from build123d import *

# Parameters (mm, degrees)
F0_W     = 15
F0_H     = 26.12
F0_W_2   = 112.35
F0_H_2   = 29.4448914682
F0_W_3   = 37.3
F1_DEPTH = 100
F2_R     = 5
F3_R     = 1
F4_R     = 0.49999
F5_R     = 3


# Not quite as in the source:
# - two fillets or chamfers of one size are made in one step
# - a fillet or chamfer is up to 0.001 mm smaller than in the source, because OpenCascade refuses the exact size
# - a feature names something its author has since deleted; it is built from what else it names


with BuildPart() as f1:
    # F0 (on Front) → F1 (new body)
    with BuildSketch(Plane.XZ):
        Polygon((0, 141.95), (0, 0), (23, 0), (23, -2), (25, -2), (25, 0), (48.9, 0), (48.9, 13.7202170637), (99.9, 13.7202170637), (99.9, 30.4702170637), (178.65, 30.4702170637), (178.65, 95.36), (28, 95.36), (28, 141.95), align=None)
        with Locations((12.5, 15.06)):
            Rectangle(F0_W, F0_H, mode=Mode.SUBTRACT)
        Polygon((25, 2), (25, 28.12), (46.9, 14.6043096234), (46.9, 2), align=None, mode=Mode.SUBTRACT)
        Polygon((97.9, 15.7202170637), (48.9, 15.7202170637), (25, 30.4702170637), (97.9, 30.4702170637), align=None, mode=Mode.SUBTRACT)
        with Locations((12.5, 46.18)):
            Rectangle(F0_W, F0_H, mode=Mode.SUBTRACT)
        with Locations((81.175, 47.1926627978)):
            Rectangle(F0_W_2, F0_H_2, mode=Mode.SUBTRACT)
        with Locations((158, 47.1926627978)):
            Rectangle(F0_W_3, F0_H_2, mode=Mode.SUBTRACT)
        with Locations((12.5, 77.3)):
            Rectangle(F0_W, F0_H, mode=Mode.SUBTRACT)
        with Locations((81.175, 78.6375542659)):
            Rectangle(F0_W_2, F0_H_2, mode=Mode.SUBTRACT)
        Polygon((25, 95.36), (5, 95.36), (5, 138.95), (17, 138.95), (17, 139.95), (25, 139.95), align=None, mode=Mode.SUBTRACT)
        with Locations((158, 78.6375542659)):
            Rectangle(F0_W_3, F0_H_2, mode=Mode.SUBTRACT)
    extrude(amount=F1_DEPTH)

    # F2
    f2_edges = [f1.edges().sort_by_distance(p)[0] for p in [
        (28, -50, 95.36),
        (25, -50, 28.12),
        (25, -50, 32.470217),
        (25, -50, 61.915109),
        (25, -50, 93.36),
        (25, -50, 63.915109),
    ]]
    fillet(f2_edges, radius=F2_R)

    # F3
    f3_edges = [f1.edges().sort_by_distance(p)[0] for p in [
        (5, -50, 64.24),
        (5, -50, 33.12),
        (5, -50, 2),
        (5, -50, 90.36),
        (5, -50, 59.24),
        (5, -50, 28.12),
        (20, -50, 28.12),
        (20, -50, 59.24),
        (20, -50, 90.36),
        (20, -50, 64.24),
        (20, -50, 33.12),
        (20, -50, 2),
        (46.9, -50, 2),
        (46.9, -50, 14.60431),
        (25, -50, 30.470217),
        (97.9, -50, 15.720217),
        (97.9, -50, 30.470217),
        (137.35, -50, 61.915109),
        (137.35, -50, 93.36),
        (137.35, -50, 63.915109),
        (137.35, -50, 32.470217),
        (176.65, -50, 32.470217),
        (176.65, -50, 63.915109),
        (139.35, -50, 63.915109),
        (139.35, -50, 61.915109),
        (139.35, -50, 93.36),
        (176.65, -50, 93.36),
        (176.65, -50, 61.915109),
        (139.35, -50, 32.470217),
        (99.9, -50, 30.470217),
        (48.9, -50, 13.720217),
        (48.9, -50, 0),
        (0, -50, 0),
        (48.9, -50, 15.720217),
        (99.9, -50, 13.720217),
        (178.65, -50, 30.470217),
        (25, -50, 139.95),
        (5, -50, 95.36),
        (5, -50, 138.95),
    ]]
    fillet(f3_edges, radius=F3_R)

    # F4 (radius 0.5 in the source; OpenCascade refuses exactly that, so slightly less here)
    f4_edges = [f1.edges().sort_by_distance(p)[0] for p in [
        (0, -50, 141.95),
        (28, -50, 141.95),
        (17, -50, 139.95),
        (17, -50, 138.95),
    ]]
    fillet(f4_edges, radius=F4_R)

    # F5
    f5_edges = [f1.edges().sort_by_distance(p)[0] for p in [
        (178.65, -50, 95.36),
        (25, -50, 95.36),
    ]]
    fillet(f5_edges, radius=F5_R)


solid = f1.part
Work out the finished part from the listing and answer in its coordinate system (mm). A direction names the side the tool comes from. Give positions to 0.01 mm unless a question says otherwise; leave off trailing zeros. Loops run counter-clockwise (first coordinate to the right, second up) from the corner with the lowest first, then second, coordinate; pieces in that order, holes last. Notation, with made-up numbers: (88, 14.25) -> (118, 14.25) arc R17 ccw to (118, 37.25) -> close; hole circle Ø2 at (89.25, -16.75). An arc over 180 degrees is marked (long way). Use a Markdown table: item, result. Add a question column.
1) The part is cut by section C-C, the plane z = 8.5. Determine the outline of the cut face in (x, y).
2) Consider line 1 along Z through (x, y) = (145.5, -70); line 2 along Z through (x, y) = (62.5, -39); line 3 along X through (y, z) = (-70, 83). Determine where each line is inside the solid, lowest interval first.
3) The part is cut by section B-B, the plane z = 72.5. Determine the outline of the cut face in (x, y).
4) For a pull along X with two mould halves and no side action, classify faces 3 (the flat face through (12, -49, 64.24)), 4 (the flat face through (99.9, -49, 22)), 5 (the flat face through (36, -49, 0)) as +X half, -X half, draft (parallel to the pull), parting line (faces both ways), or undercut.
5) The part is cut by section D-D, the plane x = 75.5. Determine the outline of the cut face in (y, z), plus the area to 3 significant figures.
6) The part is cut by section A-A, the plane x = 132.5. Determine the outline of the cut face in (y, z).
7) Each of these flat-tipped pins is pushed along its axis until it touches: P1, Ø10.5, axis at x = 13, y = -26.5, coming from the -Z side; P2, Ø2, axis at y = -77.5, z = 23, coming from the +X side; P3, Ø2, axis at x = 142.5, y = -30, coming from the -Z side. Where does it stop, or does it pass through?
8) Which of the six approach directions +Z, -Z, +X, -X, +Y, -Y give full straight-line access (tool end or side, diameter ignored) to faces 1 (the flat face through (137.35, -49, 78)), 2 (the flat face through (12, -49, 0))?
Reported:
| question | item | result |
|---|---|---|
| 1 | outline | (0, -100) -> (5, -100) -> (5, 0) -> (0, 0) -> close; (20, -100) -> (25, -100) -> (25, 0) -> (20, 0) -> close; (46.9, -100) -> (48.9, -100) -> (48.9, 0) -> (46.9, 0) -> close |
| 2 | line 1 | z = 30.47 to 32.47, 61.92 to 63.92, 93.36 to 95.36 |
| 2 | line 2 | z = 13.72 to 15.72, 30.47 to 32.47, 61.92 to 63.92, 93.36 to 95.36 |
| 2 | line 3 | x = 0 to 5, 20 to 25, 137.35 to 139.35, 176.65 to 178.65 |
| 3 | outline | (0, -100) -> (5, -100) -> (5, 0) -> (0, 0) -> close; (20, -100) -> (25, -100) -> (25, 0) -> (20, 0) -> close; (137.35, -100) -> (139.35, -100) -> (139.35, 0) -> (137.35, 0) -> close; (176.65, -100) -> (178.65, -100) -> (178.65, 0) -> (176.65, 0) -> close |
| 4 | face 3 | undercut |
| 4 | face 4 | +X half |
| 4 | face 5 | draft |
| 5 | outline | (-100, 13.72) -> (0, 13.72) -> (0, 15.72) -> (-100, 15.72) -> close; (-100, 30.47) -> (0, 30.47) -> (0, 32.47) -> (-100, 32.47) -> close; (-100, 61.92) -> (0, 61.92) -> (0, 63.92) -> (-100, 63.92) -> close; (-100, 93.36) -> (0, 93.36) -> (0, 95.36) -> (-100, 95.36) -> close |
| 5 | area | 800 mm^2 |
| 6 | outline | (-100, 30.47) -> (0, 30.47) -> (0, 32.47) -> (-100, 32.47) -> close; (-100, 61.92) -> (0, 61.92) -> (0, 63.92) -> (-100, 63.92) -> close; (-100, 93.36) -> (0, 93.36) -> (0, 95.36) -> (-100, 95.36) -> close |
| 7 | P1 | stops at z = 0 |
| 7 | P2 | stops at x = 99.9 |
| 7 | P3 | stops at z = 30.47 |
| 8 | face 1 | +Y, -Y |
| 8 | face 2 | -Z, -X, +Y, -Y |
